Check sheet for the modelled part. Datum: model origin and axes. Units: mm. Round coordinates to 2 decimals unless told otherwise and drop trailing zeros. Order: outer loops, then holes, each group sorted by start corner. A loop starts at its lowest first (then second) coordinate and runs counter-clockwise, first axis right, second up.
Q1. Cross-section at B-B on z = 8.25. Record the cut outline in (x, y).
Q2. Cross-section at C-C on x = 4. Record the cut outline in (y, z).
Q3. Mould release check, pull along X, two halves, no side actions. Record for faces 1 (the flat face through (-1, -5, 0)), 2 (the cylindrical face through (-24.3, -33.02, 7.89)), 3 (the cylindrical face through (-38.91, 12.91, 7.89)): +X half, -X half, draft (parallel to the pull), parting line (faces both ways), or undercut.
Q4. Cross-section at A-A on x = -21. Record the cut outline in (y, z), then the cut area to 3 significant figures.
Q5. Cross-section at D-D on y = -12. Record the cut outline in (x, z), then the cut area to 3 significant figures.
Q6. Depth check by flat-ended pin: P1, Ø8, axis at y = -13, z = 4.5, coming from the +X side; P2, Ø1.5, axis at y = -8.5, z = 5, coming from the -X side. Enter the tip coordinate at first touch or a pass-through.
Q7. Scan lines: probe 1 along X at (y, z) = (-9, 5.75); probe 2 along Y at (x, z) = (22, 3.25); probe 3 along X at (y, z) = (-31, 11.25). Record each from-to range of solid material in increasing order.
from build123d import *

# Parameters (mm, degrees)
F1_DEPTH = 16


with BuildPart() as f1:
    # F0 (on Top) → F1 (new body)
    with BuildSketch(Plane.XY):
        with BuildLine():
            ThreePointArc((-8.062995, 28.001486), (0, 23), (8.062995, 28.001486))
            ThreePointArc((8.062995, 28.001486), (8.762618, 29.946582), (9, 32))
            ThreePointArc((9, 32), (-2.053418, 40.762618), (-8.062995, 28.001486))
        make_face()
        with BuildLine():
            ThreePointArc((39.433809, 9.888544), (33.923096, 18.184619), (24.139393, 16.321298))
            ThreePointArc((24.139393, 16.321298), (21.8743, 7.107391), (29.122598, 0.984571))
            ThreePointArc((29.122598, 0.984571), (36.315947, 3.076756), (39.433809, 9.888544))
        make_face()
        with BuildLine():
            ThreePointArc((27.809128, -25.888544), (26.508332, -21.22783), (22.98196, -17.914368))
            ThreePointArc((22.98196, -17.914368), (13.519061, -18.607391), (9.935761, -27.392987))
            ThreePointArc((9.935761, -27.392987), (19.56401, -34.85683), (27.809128, -25.888544))
        make_face()
        with BuildLine():
            ThreePointArc((-22.98196, -17.914368), (-24.099195, -33.169697), (-9.935761, -27.392987))
            ThreePointArc((-9.935761, -27.392987), (-9.840842, -26.643425), (-9.809128, -25.888544))
            ThreePointArc((-9.809128, -25.888544), (-14.148414, -18.18934), (-22.98196, -17.914368))
        make_face()
        with BuildLine():
            ThreePointArc((-21.433809, 9.888544), (-22.137733, 13.377832), (-24.139393, 16.321298))
            ThreePointArc((-24.139393, 16.321298), (-38.993317, 12.669697), (-29.122598, 0.984571))
            ThreePointArc((-29.122598, 0.984571), (-23.622021, 4.006406), (-21.433809, 9.888544))
        make_face()
        with BuildLine():
            ThreePointArc((18.070074, -5.871323), (18.766078, -2.972255), (19, 0))
            ThreePointArc((19, 0), (16.929124, 8.625819), (11.16792, 15.371323))
            ThreePointArc((11.16792, 15.371323), (0, 19), (-11.16792, 15.371323))
            ThreePointArc((-11.16792, 15.371323), (-18.070074, 5.871323), (-18.070074, -5.871323))
            ThreePointArc((-18.070074, -5.871323), (-11.16792, -15.371323), (0, -19))
            ThreePointArc((0, -19), (11.16792, -15.371323), (18.070074, -5.871323))
        make_face()
        with BuildLine():
            ThreePointArc((22.98196, -17.914368), (18.32313, -12.791317), (18.070074, -5.871323))
            ThreePointArc((18.070074, -5.871323), (11.16792, -15.371323), (0, -19))
            ThreePointArc((0, -19), (6.503106, -21.379067), (9.935761, -27.392987))
            ThreePointArc((9.935761, -27.392987), (13.519061, -18.607391), (22.98196, -17.914368))
        make_face()
        with BuildLine():
            ThreePointArc((-9.935761, -27.392987), (-6.503106, -21.379067), (0, -19))
            ThreePointArc((0, -19), (-11.16792, -15.371323), (-18.070074, -5.871323))
            ThreePointArc((-18.070074, -5.871323), (-18.32313, -12.791317), (-22.98196, -17.914368))
            ThreePointArc((-22.98196, -17.914368), (-14.148414, -18.18934), (-9.809128, -25.888544))
            ThreePointArc((-9.809128, -25.888544), (-9.840842, -26.643425), (-9.935761, -27.392987))
        make_face()
        with BuildLine():
            ThreePointArc((-18.070074, -5.871323), (-18.070074, 5.871323), (-11.16792, 15.371323))
            ThreePointArc((-11.16792, 15.371323), (-17.827424, 13.473598), (-24.139393, 16.321298))
            ThreePointArc((-24.139393, 16.321298), (-22.137733, 13.377832), (-21.433809, 9.888544))
            ThreePointArc((-21.433809, 9.888544), (-23.622021, 4.006406), (-29.122598, 0.984571))
            ThreePointArc((-29.122598, 0.984571), (-22.342271, -0.421673), (-18.070074, -5.871323))
        make_face()
        with BuildLine():
            ThreePointArc((-11.16792, 15.371323), (0, 19), (11.16792, 15.371323))
            ThreePointArc((11.16792, 15.371323), (7.305177, 21.118458), (8.062995, 28.001486))
            ThreePointArc((8.062995, 28.001486), (0, 23), (-8.062995, 28.001486))
            ThreePointArc((-8.062995, 28.001486), (-7.305177, 21.118458), (-11.16792, 15.371323))
        make_face()
        with BuildLine():
            ThreePointArc((11.16792, 15.371323), (16.929124, 8.625819), (19, 0))
            ThreePointArc((19, 0), (18.766078, -2.972255), (18.070074, -5.871323))
            ThreePointArc((18.070074, -5.871323), (22.342271, -0.421673), (29.122598, 0.984571))
            ThreePointArc((29.122598, 0.984571), (21.8743, 7.107391), (24.139393, 16.321298))
            ThreePointArc((24.139393, 16.321298), (17.827424, 13.473598), (11.16792, 15.371323))
        make_face()
    extrude(amount=F1_DEPTH)


solid = f1.part
Results found:
1. outline: (-29.12, 0.98) arc R10.08 cw to (-18.07, -5.87) arc R10.08 cw to (-22.98, -17.91) arc R9 ccw (long way) to (-9.94, -27.39) arc R10.08 cw to (0, -19) arc R10.08 cw to (9.94, -27.39) arc R9 ccw to (27.81, -25.89) arc R9 ccw to (22.98, -17.91) arc R10.08 cw to (18.07, -5.87) arc R10.08 cw to (29.12, 0.98) arc R9 ccw to (39.43, 9.89) arc R9 ccw to (24.14, 16.32) arc R10.08 cw to (11.17, 15.37) arc R10.08 cw to (8.06, 28) arc R9 ccw to (9, 32) arc R9 ccw (long way) to (-8.06, 28) arc R10.08 cw to (-11.17, 15.37) arc R10.08 cw to (-24.14, 16.32) arc R9 ccw (long way) to start
2. outline: (-19.83, 0) - (40.06, 0) - (40.06, 16) - (-19.83, 16) - close
3. face 1: draft
3. face 2: undercut
3. face 3: undercut
4. outline: (-34.62, 0) - (-16.55, 0) - (-16.55, 16) - (-34.62, 16) - close; (-1.42, 0) - (14.24, 0) - (14.24, 16) - (-1.42, 16) - close
4. area: 539 mm2
5. outline: (-18.04, 0) - (18.04, 0) - (18.04, 16) - (-18.04, 16) - close
5. area: 577 mm2
6. P1: stops at x = 21.55
6. P2: stops at x = -17.65
7. probe 1: x = -17.58 to 17.58
7. probe 2: y = -34.3 to -17.33, -0.64 to 14.72
7. probe 3: x = -26.22 to -11.4, 11.4 to 26.22
